Model file for the job. Use its own axes, mm. A direction names the side the tool comes from. Coordinates: 2 decimals unless noted, no trailing zeros. Write each loop counter-clockwise with the first axis right and the second up, starting at its lowest first coordinate (ties: lowest second). Pieces come first, ordered by that corner, then holes. Notation, with made-up numbers: M 2,66.25 L 48,66.25 A24 ccw 48,88.25 Z; hole C 14,43 d3. An arc over 180 degrees is marked long. Put each result on its own line as item: value. Start each with the question number.
Q1. Cut at C-C (y = 50). Write the cut outline in (x, z), then the cut area to 3 significant figures.
Q2. Cut at B-B (x = -3.25). Write the cut outline in (y, z), then the cut area to 3 significant figures.
Q3. Which spindle directions (+Z, -Z, +X, -X, +Y, -Y) get a long thin tool onto all of the face, cutting with end or side? Do faces 1 (the cylindrical face through (-16.6, 48.8, -17.66)), 2 (the flat face through (-30.3, 48.5, -22.6)), 3 (the cylindrical face through (7.252, 47.941, -31.787)), 4 (the cylindrical face through (-7.14, 47.94, -23.47)), 5 (the flat face through (6.5, 48, -27)). Say none if no direction does.
Q4. Drop flat-ended pins along their axis: pin 1 (1 mm diameter, centred on x = 0.5, z = -29.5, fed in from -Y); pin 2 (2.5 mm diameter, centred on x = 3.25, z = -27.2, fed in from +Y); pin 3 (1.5 mm diameter, centred on x = -3.25, z = -27.2, fed in from +Y); pin 4 (2.5 mm diameter, centred on y = 49, z = -28, fed in from -X). Give the stop position or say it passes through.
Q5. Pull direction Z, two halves, no side cores. Call faces 6 (the cylindrical face through (37.5, 48.7, -25.16)), 7 (the cylindrical face through (31.038, 46.726, -23.004)), 8 (the flat face through (0, 52.5, -25)): pulls with the +Z half, pulls with the -Z half, needs draft (parallel to the pull), parting line crosses it, or undercut.
Q6. Drill centre lines: line 1 along X through (y, z) = (50.55, -25); line 2 along X through (y, z) = (51.75, -25); line 3 along X through (y, z) = (47.2, -25). Where is each one in solid material? Low to high.
Q7. Cut at A-A (y = 46). Write the cut outline in (x, z).
```python
from build123d import *

# Parameters (mm, degrees)
SKETCH1_R           = 2.25
BOSS_EXTRUDE1_DEPTH = 7.5
SKETCH2_R           = 0.85
CUT_EXTRUDE1_DEPTH  = 8.5
SKETCH3_R           = 0.85
BOSS_EXTRUDE2_DEPTH = 1.7
SKETCH4_W           = 13.2
SKETCH4_H           = 9.425338572
CUT_EXTRUDE2_DEPTH  = 5.8
FILLET1_R           = 2.5
SKETCH5_R           = 3.75
CUT_EXTRUDE3_DEPTH  = 4


with BuildPart() as part:
    # Sketch1 → Boss-Extrude1 (new body)
    with BuildSketch(Plane(origin=(0, 45, 0), x_dir=(1, 0, 0), z_dir=(0, 1, 0))):
        with BuildLine():
            Line((-16.524067706, 17.5), (-30.2, 17.5))
            ThreePointArc((-30.2, 17.5), (-37.7, 25), (-30.2, 32.5))
            Line((-30.2, 32.5), (30, 32.5))
            ThreePointArc((30, 32.5), (37.5, 25), (30, 17.5))
            Line((30, 17.5), (16.324067706, 17.5))
            ThreePointArc((16.324067706, 17.5), (-0.1, 24), (-16.524067706, 17.5))
        make_face()
        with Locations((-30.2, 25)):
            Circle(SKETCH1_R, mode=Mode.SUBTRACT)
        with Locations((30, 25)):
            Circle(SKETCH1_R, mode=Mode.SUBTRACT)
    extrude(amount=BOSS_EXTRUDE1_DEPTH)

    # Sketch2 → Cut-Extrude1 (cut, through all)
    with BuildSketch(Plane.XZ.offset(-45)):
        with Locations((-3.25, -27.2)):
            Circle(SKETCH2_R)
        with Locations((3.25, -27.2)):
            Circle(SKETCH2_R)
    extrude(amount=-CUT_EXTRUDE1_DEPTH, mode=Mode.SUBTRACT)

    # Sketch3 → Boss-Extrude2 (add)
    with BuildSketch(Plane.XZ.offset(-52.5)):
        with BuildLine():
            Line((-3.25, -24.7), (3.25, -24.7))
            ThreePointArc((3.25, -24.7), (5.75, -27.2), (3.25, -29.7))
            Line((3.25, -29.7), (-3.25, -29.7))
            ThreePointArc((-3.25, -29.7), (-5.75, -27.2), (-3.25, -24.7))
        make_face()
        with Locations((3.25, -27.2)):
            Circle(SKETCH3_R, mode=Mode.SUBTRACT)
        with Locations((-3.25, -27.2)):
            Circle(SKETCH3_R, mode=Mode.SUBTRACT)
    extrude(amount=BOSS_EXTRUDE2_DEPTH)

    # Sketch4 → Cut-Extrude2 (cut)
    with BuildSketch(Plane(origin=(0, 45, 0), x_dir=(1, 0, 0), z_dir=(0, 1, 0))):
        with Locations((-0.1, 27.787330714)):
            Rectangle(SKETCH4_W, SKETCH4_H)
    extrude(amount=CUT_EXTRUDE2_DEPTH, mode=Mode.SUBTRACT)

    # Fillet1
    fillet1_edges = [part.edges().sort_by_distance(p)[0] for p in [
        (-16.524067706, 48.75, -17.5),
        (16.324067706, 48.75, -17.5),
        (-6.7, 47.9, -32.5),
        (-6.7, 47.9, -23.074661428),
        (6.5, 47.9, -23.074661428),
        (6.5, 47.9, -32.5),
    ]]
    fillet(fillet1_edges, radius=FILLET1_R)

    # Sketch5 → Cut-Extrude3 (cut)
    with BuildSketch(Plane(origin=(0, 52.5, 0), x_dir=(1, 0, 0), z_dir=(0, 1, 0))):
        with Locations((-30.2, 25)):
            Circle(SKETCH5_R)
        with Locations((30, 25)):
            Circle(SKETCH5_R)
    extrude(amount=-CUT_EXTRUDE3_DEPTH, mode=Mode.SUBTRACT)


solid = part.part
```
Computed values:
1. outline: M -30.2,-32.5 L -9.2,-32.5 A2.5 ccw -6.7,-30 L -6.7,-24.89 A2.5 ccw -8.34,-22.54 A24 cw -15.85,-18.11 A2.5 ccw -17.49,-17.5 L -30.2,-17.5 A7.5 ccw Z; M 6.5,-30 A2.5 ccw 9,-32.5 L 30,-32.5 A7.5 ccw 30,-17.5 L 17.29,-17.5 A2.5 ccw 15.65,-18.11 A24 cw 8.14,-22.54 A2.5 ccw 6.5,-24.89 Z; hole C -30.2,-25 d7.5; hole C 30,-25 d7.5
1. area: 724 mm2
2. outline: M 50.8,-32.5 L 52.5,-32.5 L 52.5,-28.05 L 50.8,-28.05 Z; M 50.8,-26.35 L 52.5,-26.35 L 52.5,-23.79 L 50.8,-23.79 Z
2. area: 11.9 mm2
3. face 1: +Z, +Y, -Y
3. face 2: +Y
3. face 3: -Z, -Y
3. face 4: +Z, -Y
3. face 5: +Z, -Z, -Y
4. pin 1: y = 50.8
4. pin 2: y = 52.5
4. pin 3: through
4. pin 4: x = -37.49
5. face 6: parting line crosses it
5. face 7: undercut
5. face 8: needs draft
6. line 1: -37.7 to -33.95, -26.45 to -6.7, 6.5 to 26.25, 33.75 to 37.5
6. line 2: -37.7 to -33.95, -26.45 to 26.25, 33.75 to 37.5
6. line 3: -37.7 to -32.45, -27.95 to -6.7, 6.5 to 27.75, 32.25 to 37.5
7. outline: M -30.2,-32.5 L -9.2,-32.5 A2.5 ccw -6.7,-30 L -6.7,-24.89 A2.5 ccw -8.34,-22.54 A24 cw -15.85,-18.11 A2.5 ccw -17.49,-17.5 L -30.2,-17.5 A7.5 ccw Z; M 6.5,-30 A2.5 ccw 9,-32.5 L 30,-32.5 A7.5 ccw 30,-17.5 L 17.29,-17.5 A2.5 ccw 15.65,-18.11 A24 cw 8.14,-22.54 A2.5 ccw 6.5,-24.89 Z; hole C -30.2,-25 d4.5; hole C 30,-25 d4.5
